Design review of the part built by this model. Coordinates are the model's own, in mm. Give positions to 0.01 mm unless a question says otherwise; leave off trailing zeros. Order: outer loops, then holes, each group sorted by start corner. A loop starts at its lowest first (then second) coordinate and runs counter-clockwise, first axis right, second up.
Autodesk Inventor part; units mm, degrees
ref_plane "YZ Plane" through (0, 0, 0) normal (1, 0, 0) x (0, 1, 0)
ref_plane "XZ Plane" through (0, 0, 0) normal (0, 1, 0) x (-1, 0, 0)
ref_plane "XY Plane" through (0, 0, 0) normal (0, 0, 1) x (1, 0, 0)
sketch "スケッチ1" plane through (0, 0, 0) normal (0, 1, 0) x (-1, 0, 0)
  circle A0 centre (0, 0) radius 9.15
  circle A1 centre (0, 0) radius 16
  dimension "d0" = 18.3
  dimension "d1" = 32
extrude "押し出し1" add sketch "スケッチ1" along normal blind 1.1
sketch "スケッチ2" plane through (0, 1.1, 0) normal (0, 1, 0) x (1, 0, 0)
  circle A0 centre (0, 0) radius 12.5 construction
  point P0 (-12.5, 0)
  point P1 (0, 12.5)
  point P2 (12.5, 0)
  point P3 (0, -12.5)
  dimension "d4" = 25
hole "穴1" at (-12.5, 1.1, 0) at (0, 1.1, -12.5) at (12.5, 1.1, 0) at (0, 1.1, 12.5) direction (0, -1, 0) diameter 3.5 end through all
properties part number "shoulder2_shaftholder_spacer"
1. For line 1 along Z through (x, y) = (0, 0.85); line 2 along Z through (x, y) = (-1, 0.2); line 3 along X through (y, z) = (0.5, 12.5), list the stretches that pass through material, from the lowest coordinate up.
Recorded:
line 1: z = -16 to -14.25, -10.75 to -9.15, 9.15 to 10.75, 14.25 to 16
line 2: z = -15.97 to -13.94, -11.06 to -9.1, 9.1 to 11.06, 13.94 to 15.97
line 3: x = -9.99 to -1.75, 1.75 to 9.99
2. Take a section at C-C (z = 3). State the section outline as (x, y) points.
Recorded:
outline: (-15.72, 0) - (-8.64, 0) - (-8.64, 1.1) - (-15.72, 1.1) - close; (8.64, 0) - (15.72, 0) - (15.72, 1.1) - (8.64, 1.1) - close
3. Draft analysis for pull direction Z (two halves, no side actions). For faces 1 (the face through (-4.919, 0.542, -7.715)), 2 (the face through (-7, 1.1, -7)), 3 (the face through (3.47, 0.54, 15.62)), state which applies: pulls with the +Z half, pulls with the -Z half, needs draft (parallel to the pull), parting line crosses it, or undercut.
Recorded:
face 1: undercut
face 2: needs draft
face 3: parting line crosses it
4. Take a section at B-B (x = -12.5). State the section outline as (y, z) points.
Recorded:
outline: (0, -9.99) - (1.1, -9.99) - (1.1, -1.75) - (0, -1.75) - close; (0, 1.75) - (1.1, 1.75) - (1.1, 9.99) - (0, 9.99) - close
5. Take a section at A-A (y = 0.55). State the section outline as (x, z) points.
Recorded:
outline: circle Ø32 at (0, 0); hole circle Ø3.5 at (-12.5, 0); hole circle Ø18.3 at (0, 0); hole circle Ø3.5 at (0, -12.5); hole circle Ø3.5 at (0, 12.5); hole circle Ø3.5 at (12.5, 0)
